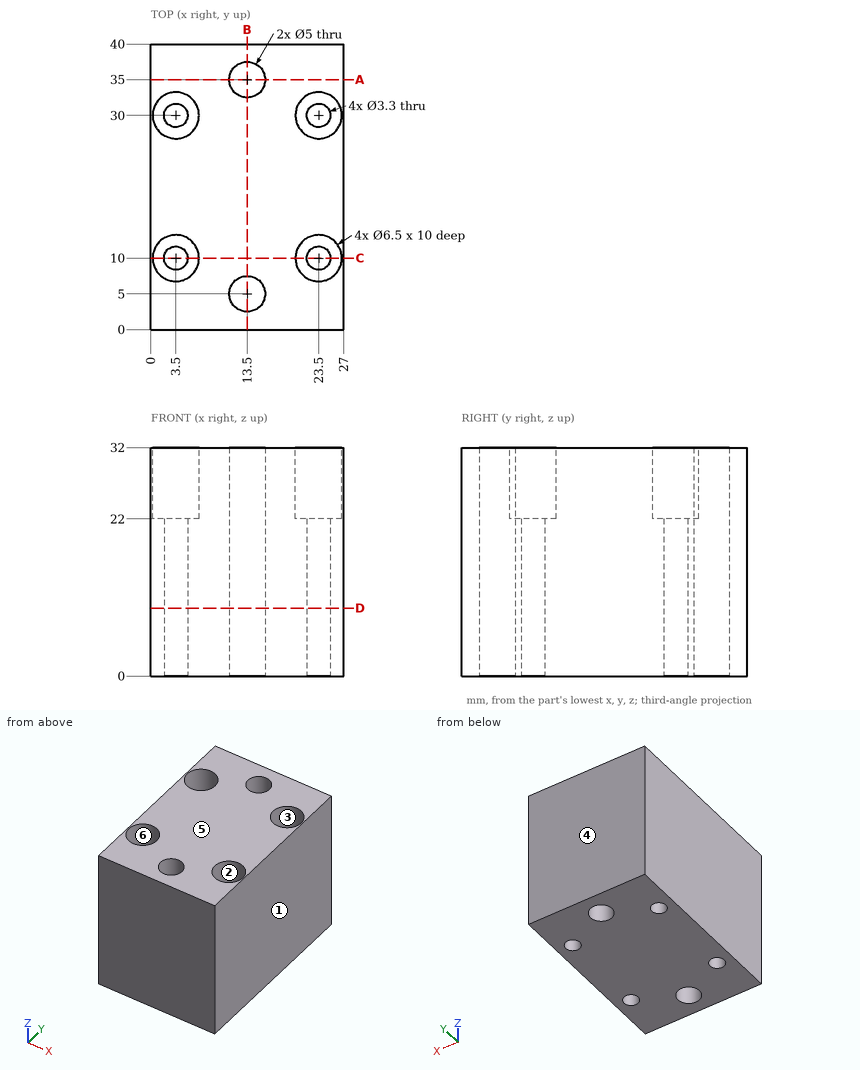
Drawing for the job (mm, zero at the part's lowest x, y, z). A direction names the side the tool comes from. Coordinates: 2 decimals unless noted, no trailing zeros. Order: outer loops, then holes, each group sorted by start corner. A loop starts at its lowest first (then second) coordinate and runs counter-clockwise, first axis right, second up.
Item 1: Two-plate mould, pull along Y, no slides. Class the marked faces 1, 2, 3 and 4: +Y half, -Y half, draft (parallel to the pull), parting line (faces both ways), or undercut.
Check sheet entries:
face 1: draft
face 2: undercut
face 3: undercut
face 4: +Y half
Item 2: Band-saw the part on D-D on z = 9.5. List the corners of the cut face in (x, y).
Check sheet entries:
outline: (0, 0) - (27, 0) - (27, 40) - (0, 40) - close; hole circle Ø3.3 at (3.5, 10); hole circle Ø3.3 at (3.5, 30); hole circle Ø5 at (13.5, 5); hole circle Ø5 at (13.5, 35); hole circle Ø3.3 at (23.5, 10); hole circle Ø3.3 at (23.5, 30)
Item 3: Band-saw the part on B-B on x = 13.5. List the corners of the cut face in (y, z).
Check sheet entries:
outline: (0, 0) - (2.5, 0) - (2.5, 32) - (0, 32) - close; (7.5, 0) - (32.5, 0) - (32.5, 32) - (7.5, 32) - close; (37.5, 0) - (40, 0) - (40, 32) - (37.5, 32) - close
Item 4: 3-axis set-ups, long thin cutter, end or side, ignore diameter. For the marked faces 5 and 6: which of +Z, -Z, +X, -X, +Y, -Y reach the whole face in a straight line?
Check sheet entries:
face 5: +Z, +X, -X, +Y, -Y
face 6: +Z
Item 5: Band-saw the part on C-C on y = 10. List the corners of the cut face in (x, z).
Check sheet entries:
outline: (0, 0) - (1.85, 0) - (1.85, 22) - (0.25, 22) - (0.25, 32) - (0, 32) - close; (5.15, 0) - (21.85, 0) - (21.85, 22) - (20.25, 22) - (20.25, 32) - (6.75, 32) - (6.75, 22) - (5.15, 22) - close; (25.15, 0) - (27, 0) - (27, 32) - (26.75, 32) - (26.75, 22) - (25.15, 22) - close
Item 6: Pin check, flat tips, straight feed: pin 1 Ø5 at (x, y) = (4, 9.5) entering from +Z; pin 2 Ø6.5 at (x, y) = (13.5, 5) entering from +Z. Stop position of each tip, or through.
Check sheet entries:
pin 1: stops at z = 22
pin 2: stops at z = 32
Item 7: Drill centre lines: L1, parallel to Y at x = 3.5, z = 27.75; L2, parallel to Y at x = 13.5, z = 17.5; L3, parallel to X at y = 11.5, z = 9.5. Where is each one in solid material? Low to high.
Check sheet entries:
L1: y = 0 to 6.75, 13.25 to 26.75, 33.25 to 40
L2: y = 0 to 2.5, 7.5 to 32.5, 37.5 to 40
L3: x = 0 to 2.81, 4.19 to 22.81, 24.19 to 27
Item 8: Band-saw the part on A-A on y = 35. List the corners of the cut face in (x, z).
Check sheet entries:
outline: (0, 0) - (11, 0) - (11, 32) - (0, 32) - close; (16, 0) - (27, 0) - (27, 32) - (16, 32) - close
